Build history of the part. All positions in model axes, mm. Face numbers are marked on the shaded views. A direction names the side the tool comes from. Give positions to 0.01 mm unless a question says otherwise; leave off trailing zeros. Write each loop counter-clockwise with the first axis right and the second up, starting at its lowest first coordinate (ties: lowest second). Pieces come first, ordered by that corner, then holes.
from build123d import *

# Parameters (mm, degrees)
F0_W           = 85.852
F0_H           = 12.7
F1_DEPTH       = 50.8
F3_D           = 7.874
F3_CBORE_D     = 12.7
F3_CBORE_DEPTH = 6.35
F4_DEPTH       = 25.4
F5_W           = 19.05
F5_H           = 53.848
F6_DEPTH       = 12.7
F7_W           = 12.7
F7_H           = 6.096
F8_DEPTH       = 53.848


with BuildPart() as f1:
    # F0 (on Front) → F1 (new body)
    with BuildSketch(Plane.XZ):
        with Locations((42.926, 6.35)):
            Rectangle(F0_W, F0_H)
        Polygon((85.852, 12.7), (85.852, 0), (135.4230137883, 49.5710137883), (129.0730137883, 55.9210137883), align=None)
    extrude(amount=F1_DEPTH)

    # F3 (through all)
    with Locations(Plane.XY.offset(12.7)):
        with Locations((15.748, -12.7), (15.748, -38.1), (70.104, -38.1), (70.104, -12.7)):
            CounterBoreHole(F3_D / 2, F3_CBORE_D / 2, F3_CBORE_DEPTH)

    # F0 (on Front) → F4 (join)
    with BuildSketch(Plane.XZ):
        Polygon((85.852, 12.7), (85.852, 0), (135.4230137883, 49.5710137883), (129.0730137883, 55.9210137883), align=None)
    extrude(amount=F4_DEPTH)

    # F5 (on face) → F6 (join)
    with BuildSketch(Plane(origin=(42.926, 0, -42.926), x_dir=(0, 1, 0), z_dir=(0.7071067812, 0, -0.7071067812))):
        with Locations((-9.525, 103.8865313784)):
            Rectangle(F5_W, F5_H)
        with Locations((-41.275, 103.8865313784)):
            Rectangle(F5_W, F5_H)
    extrude(amount=F6_DEPTH)

    # F7 (on face) → F8 (cut)
    with BuildSketch(Plane(origin=(92.4970137883, 0, 92.4970137883), x_dir=(0, 1, 0), z_dir=(0.7071067812, 0, 0.7071067812))):
        with Locations((-12.7, -63.7545313784)):
            Rectangle(F7_W, F7_H)
        with Locations((-38.1, -63.7545313784)):
            Rectangle(F7_W, F7_H)
    extrude(amount=-F8_DEPTH, mode=Mode.SUBTRACT)


solid = f1.part
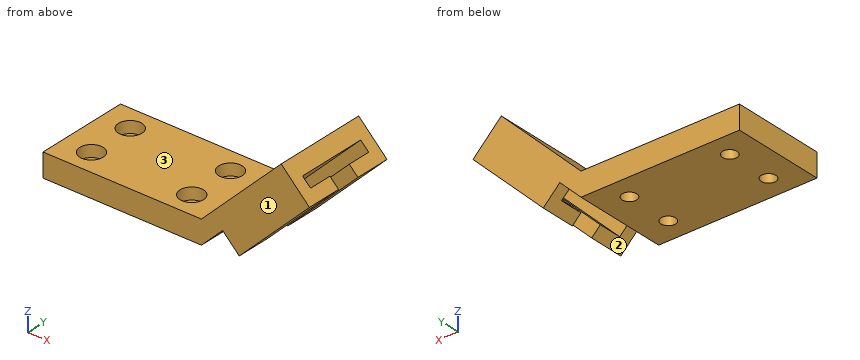
1. Saw through at C-C on y = -46.5. Give the cut face in (x, z).
2. Drill centre lines: line 1 along Y through (x, z) = (124.5, 22); line 2 along X through (y, z) = (-38, 4); line 3 along X through (y, z) = (-12, 1). Where is each one in solid material? Low to high.
3. Saw through at B-B on z = 5. Give the cut face in (x, y).
4. Drop flat-ended pins along their axis: pin 1 (12.5 mm diameter, centred on x = 70.104, y = -38.1, fed in from +Z); pin 2 (15 mm diameter, centred on x = 31.5, y = -15, fed in from +Z); pin 3 (4 mm diameter, centred on y = -26, z = 38.5, fed in from +X). Give the stop position or say it passes through.
5. Saw through at A-A on y = -38.1. Count the separate pieces of the cut face and the enclosed holes in it, plus the area to 3 significant figures.
6. 3-axis set-ups, long thin cutter, end or side, ignore diameter. For the marked faces 1, 2 and 3: which of +Z, -Z, +X, -X, +Y, -Y reach the whole face in a straight line?
7. Saw through at D-D on x = 100. Give the cut face in (y, z).
Outcome:
1. outline: (0, 0) - (85.85, 0) - (97.35, 11.49) - (106.33, 2.51) - (144.4, 40.59) - (129.07, 55.92) - (85.85, 12.7) - (0, 12.7) - close
2. line 1: y = -50.8 to -31.75, -19.05 to 0
2. line 2: x = 0 to 11.81, 19.68 to 66.17, 74.04 to 89.85, 104.84 to 107.81
2. line 3: x = 0 to 11.87, 19.62 to 66.23, 73.98 to 86.85
3. outline: (0, -50.8) - (90.85, -50.8) - (90.85, 0) - (0, 0) - close; (103.84, -50.8) - (108.81, -50.8) - (108.81, -31.75) - (103.84, -31.75) - close; (103.84, -19.05) - (108.81, -19.05) - (108.81, 0) - (103.84, 0) - close; hole circle Ø7.87 at (15.75, -38.1); hole circle Ø7.87 at (15.75, -12.7); hole circle Ø7.87 at (70.1, -38.1); hole circle Ø7.87 at (70.1, -12.7)
4. pin 1: stops at z = 6.35
4. pin 2: stops at z = 12.7
4. pin 3: stops at x = 126.35
5. separate pieces: 4
5. enclosed holes: 0
5. area: 1,770 mm2
6. face 1: +Z, -Z, +X, -X, -Y
6. face 2: -Z, +Y, -Y
6. face 3: +Z, -X, +Y, -Y
7. outline: (-50.8, 8.84) - (-44.45, 8.84) - (-44.45, 14.15) - (-6.35, 14.15) - (-6.35, 8.84) - (0, 8.84) - (0, 26.85) - (-50.8, 26.85) - close
